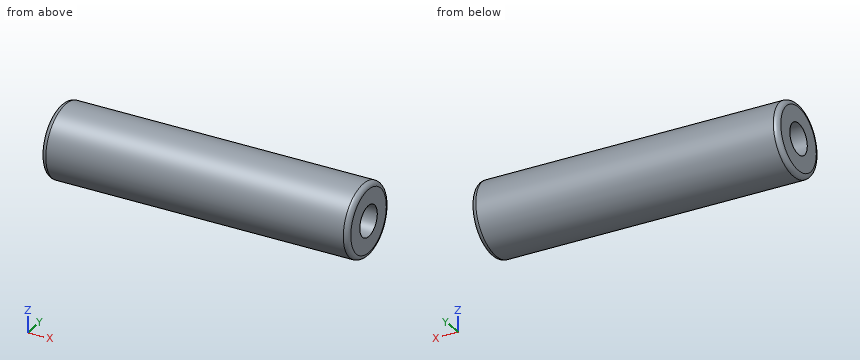
from build123d import *

# Parameters (mm, degrees)
SKETCH1_R           = 4.7625
BOSS_EXTRUDE1_DEPTH = 20.32
SKETCH3_R           = 2.032
CUT_EXTRUDE1_DEPTH  = 42.194325004
FILLET1_R           = 0.635


with BuildPart() as part:
    # Sketch1 → Boss-Extrude1 (new, symmetric)
    with BuildSketch(Plane(origin=(0, 0, 0), x_dir=(0, 0, -1), z_dir=(1, 0, 0))):
        Circle(SKETCH1_R)
    extrude(amount=BOSS_EXTRUDE1_DEPTH, both=True)

    # Sketch3 → Cut-Extrude1 (cut, through all)
    with BuildSketch(Plane(origin=(20.32, 0, 0), x_dir=(0, 0, -1), z_dir=(1, 0, 0))):
        Circle(SKETCH3_R)
    extrude(amount=-CUT_EXTRUDE1_DEPTH, mode=Mode.SUBTRACT)

    # Fillet1
    fillet1_edges = [part.edges().sort_by_distance(p)[0] for p in [
        (-20.32, 0, 4.7625),
        (20.32, 0, 4.7625),
    ]]
    fillet(fillet1_edges, radius=FILLET1_R)


solid = part.part
Could you check a few things on this model? Use its own coordinates, in mm. Give positions to 0.01 mm unless a question says otherwise; leave off trailing zeros. Order: outer loops, then holes, each group sorted by start corner. A loop starts at its lowest first (then second) coordinate and runs counter-clockwise, first axis right, second up. Notation, with made-up numbers: (-34.75, 82.25) - (17.25, 82.25) arc R16 ccw to (17.25, 97.25) - close; hole circle Ø2 at (51.25, 53). An arc over 180 degrees is marked (long way). Return JSON: item names as keys, results as strings. Group by question number.
Q1. Please list where these lines run through material, in increasing order: line 1 along Y through (x, z) = (-5, 0); line 2 along Y through (x, z) = (-11.5, 1); line 3 along Z through (x, y) = (9, 0.5). Write a range as [from, to].
Q2. Will these pins go through, and if not, where does the flat tip stop? pin 1 Ø1 at (x, z) = (-11, -3.5) entering from +Y; pin 2 Ø3 at (x, y) = (-11.5, -3.5) entering from +Z.
Q3. Suppose I cut it at C-C, the plane x = 15. Please give me the cut outline in (y, z) (1 decimal).
Q4. Suppose I cut it at A-A, the plane y = 0. Please give me the cut outline in (x, z) (1 decimal), and give its area (3 significant figures).
Resolved:
{
 "1": {"line 1": "y = [-4.76, -2.03], [2.03, 4.76]", "line 2": "y = [-4.66, -1.77], [1.77, 4.66]", "line 3": "z = [-4.74, -1.97], [1.97, 4.74]"},
 "2": {"pin 1": "stops at y = 3.7", "pin 2": "stops at z = 4.32"},
 "3": {"outline": "circle Ø9.5 at (0, 0); hole circle Ø4.1 at (0, 0)"},
 "4": {"outline": "(-20.3, -4.1) arc R0.6 ccw to (-19.7, -4.8) - (19.7, -4.8) arc R0.6 ccw to (20.3, -4.1) - (20.3, -2) - (-20.3, -2) - close; (-20.3, 2) - (20.3, 2) - (20.3, 4.1) arc R0.6 ccw to (19.7, 4.8) - (-19.7, 4.8) arc R0.6 ccw to (-20.3, 4.1) - close", "area": "222 mm2"}
}
